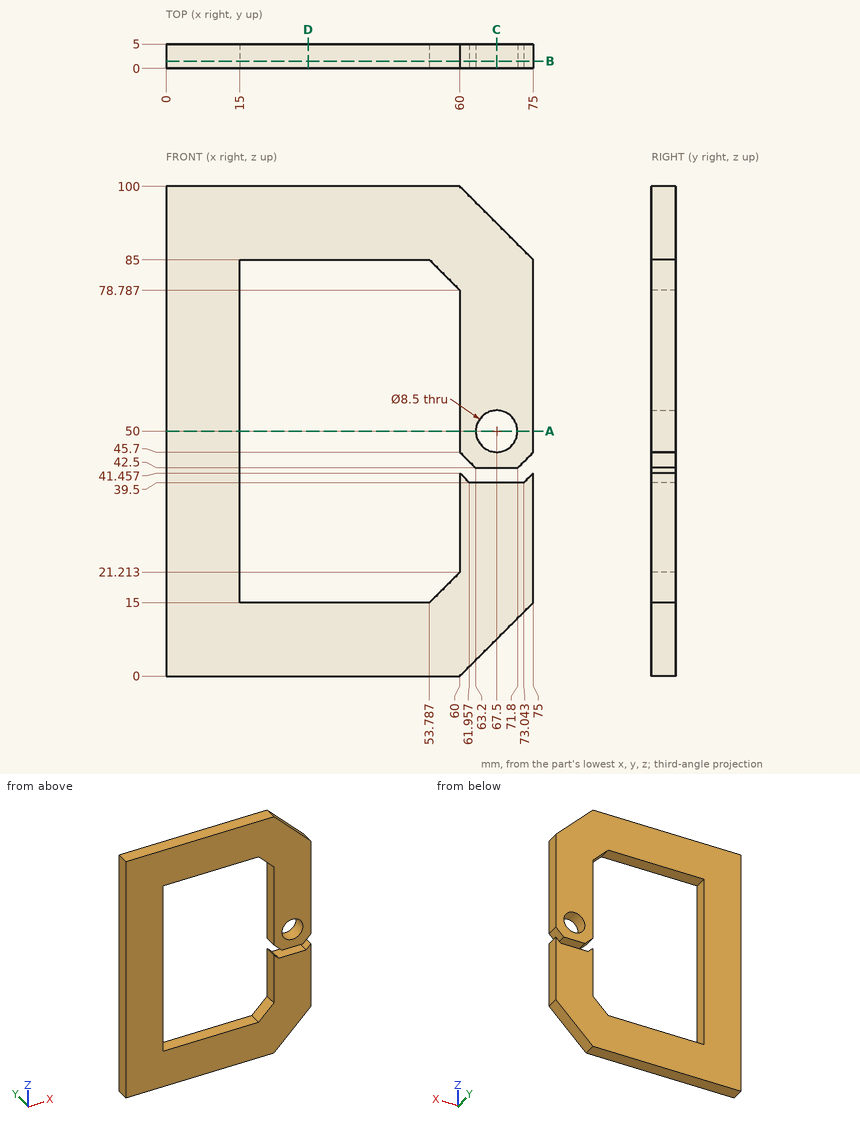
Drawing for the job (mm, zero at the part's lowest x, y, z). Give positions to 0.01 mm unless a question says otherwise; leave off trailing zeros. Order: outer loops, then holes, each group sorted by start corner. A loop starts at its lowest first (then second) coordinate and runs counter-clockwise, first axis right, second up. Notation, with made-up numbers: M 40.5,35.25 L 98.5,35.25 A26 cw 98.5,72.25 Z; hole C -23,78.25 d7. An arc over 180 degrees is marked long. Put each result on its own line as item: value. Start each with the question number.
(1) Drill centre lines: line 1 along Z through (x, y) = (53.5, 2.5); line 2 along X through (y, z) = (1.65, 52.5); line 3 along X through (y, z) = (3.7, 26). Where is each one in solid material? Low to high.
(2) Saw through at B-B, the plane y = 1.5. Write the cut outline in (x, z), then the cut area to 3 significant figures.
(3) Saw through at D-D, the plane x = 29. Write the cut outline in (y, z).
(4) Flat gauge pins, fed straight in: pin 1 Ø2.5 at (x, y) = (68, 2.5) entering from -Z; pin 2 Ø2.5 at (x, y) = (67, 3.5) entering from +Z. Where does each tip first touch, or does it go through?
(5) Saw through at C-C, the plane x = 67.5. Write the cut outline in (y, z).
(6) Saw through at A-A, the plane z = 50. Write the cut outline in (x, y).
Check result:
1. line 1: z = 0 to 15, 85 to 100
1. line 2: x = 0 to 15, 60 to 64.06, 70.94 to 75
1. line 3: x = 0 to 15, 60 to 75
2. outline: M 0,0 L 60,0 L 75,15 L 75,41.46 L 73.04,39.5 L 61.96,39.5 L 60,41.46 L 60,21.21 L 53.79,15 L 15,15 L 15,85 L 53.79,85 L 60,78.79 L 60,45.7 L 63.2,42.5 L 71.8,42.5 L 75,45.7 L 75,85 L 60,100 L 0,100 Z; hole C 67.5,50 d8.5
2. area: 4,060 mm2
3. outline: M 0,0 L 5,0 L 5,15 L 0,15 Z; M 0,85 L 5,85 L 5,100 L 0,100 Z
4. pin 1: stops at z = 6.75
4. pin 2: stops at z = 94.25
5. outline: M 0,7.5 L 5,7.5 L 5,39.5 L 0,39.5 Z; M 0,42.5 L 5,42.5 L 5,45.75 L 0,45.75 Z; M 0,54.25 L 5,54.25 L 5,92.5 L 0,92.5 Z
6. outline: M 0,0 L 15,0 L 15,5 L 0,5 Z; M 60,0 L 63.25,0 L 63.25,5 L 60,5 Z; M 71.75,0 L 75,0 L 75,5 L 71.75,5 Z
